```python
from build123d import *


with BuildPart() as part:
    # Sketch1 → Revolve1 (revolve)
    with BuildSketch(Plane.XY, mode=Mode.PRIVATE) as revolve1_sk:
        with BuildLine():
            Line((1.795946189, 30.1625), (1.795946189, 40.64))
            ThreePointArc((1.795946189, 40.64), (1.981933383, 41.089012806), (2.430946189, 41.275))
            Line((2.430946189, 41.275), (10.685946189, 41.275))
            Line((10.685946189, 41.275), (10.685946189, 45.7835))
            ThreePointArc((10.685946189, 45.7835), (10.760341067, 45.963105122), (10.939946189, 46.0375))
            Line((10.939946189, 46.0375), (12.324748868, 46.0375))
            ThreePointArc((12.324748868, 46.0375), (12.50435399, 46.111894878), (12.578748868, 46.2915))
            Line((12.578748868, 46.2915), (12.578748868, 48.0695))
            ThreePointArc((12.578748868, 48.0695), (12.764736062, 48.518512806), (13.213748868, 48.7045))
            Line((13.213748868, 48.7045), (28.211946189, 48.7045))
            ThreePointArc((28.211946189, 48.7045), (28.660958995, 48.518512806), (28.846946189, 48.0695))
            Line((28.846946189, 48.0695), (28.846946189, 30.1625))
            Line((28.846946189, 30.1625), (1.795946189, 30.1625))
        make_face()
    revolve(revolve1_sk.sketch.rotate(Axis((0, 0, 0), (1, 0, 0)), 90), axis=Axis((0, 0, 0), (1, 0, 0)))


solid = part.part
```
For this review, take the finished solid that the model builds, in its own axes (mm). A direction names the side the tool comes from. Round coordinates to 2 decimals unless told otherwise and drop trailing zeros. Write each loop counter-clockwise with the first axis right and the second up, starting at its lowest first coordinate (ties: lowest second). Pieces come first, ordered by that corner, then holes. Notation, with made-up numbers: (6, 5) -> (45, 5) arc R19 ccw to (45, 42) -> close; hole circle Ø11 at (46.5, -34.75). An arc over 180 degrees is marked (long way). Use one line per item in the form item = value.
Q1. Consider section C-C (x = 25). State the section outline as (y, z) points (1 decimal), then the cut area to 3 significant figures.
Resolved:
outline = circle Ø97.4 at (0, 0); hole circle Ø60.3 at (0, 0)
area = 4,590 mm²
Q2. The part is to be moulded in two halves that separate along Z. For faces 1 (the flat face through (12.579, -39.4, 25.1)), 2 (the cylindrical face through (11.642, 44.943, -9.98)), 3 (the cylindrical face through (15.132, -1.326, -30.133)), say which applies: released by +Z, released by -Z, zero draft, split by the parting line, or undercut.
Resolved:
face_1 = zero draft
face_2 = split by the parting line
face_3 = undercut
Q3. Clearance check with flat-ended pins moving along their axes: pin 1 Ø10 at (x, y) = (23, 4) entering from -Z; pin 2 Ø1.5 at (x, y) = (13, -10) entering from -Z; pin 3 Ø3 at (x, y) = (8, 22.5) entering from -Z; pin 4 Ø6 at (y, z) = (23.5, 13) entering from -X. State where each tip first meets the part, or that it passes through.
Resolved:
pin_1 = -48.7
pin_2 = -47.81
pin_3 = -35.53
pin_4 = through
Q4. To check wall thickness, follow probe 1 along Y at (x, z) = (9.75, 0) (1 decimal); probe 2 along Y at (x, z) = (13.5, 0); probe 3 along X at (y, z) = (11.5, -42.5). State the ranges of each line that lie inside material, in increasing order. Write a range as from..to.
Resolved:
probe_1 = -41.3..-30.2, 30.2..41.3
probe_2 = -48.7..-30.16, 30.16..48.7
probe_3 = 10.69..28.85
Q5. Machinability: for faces 4 (the cylindrical face through (20.818, -14.63, 46.455)), 5 (the cylindrical face through (6.616, -40.924, -5.373)), which of the approach directions +Z, -Z, +X, -X, +Y, -Y give a long, thin tool a straight path to every point of the face, cutting with its end or side? Answer none if there is none.
Resolved:
face_4 = +X, -X
face_5 = -X
